from build123d import *

# Parameters (mm, degrees)
BALL_CUT_PATTERN_COUNT      = 3
M3X0_5_TAPPED_HOLE1_REACH   = 23.674
M3X0_5_TAPPED_HOLE1_BORE_R  = 1.25
SET_SCREW_PATTERN_OUTLINE_W = 1.25
SET_SCREW_PATTERN_OUTLINE_H = 2.885095828


# Read off the part's stored shape, not the designer's step: Set Screw Pattern
with BuildPart() as part:
    # Body Sketch → Body Revolve (revolve)
    with BuildSketch(Plane(origin=(-33.219700818, 0, -2.434260963), x_dir=(-1, 0, 0), z_dir=(0, 1, 0)), mode=Mode.PRIVATE) as body_revolve_sk:
        Polygon((-35.719700818, 24.434260963), (-38.269700818, 24.434260963), (-38.269700818, 10.434260963), (-38.169700818, 10.434260963), (-38.169700818, 3.434260963), (-38.269700818, 3.434260963), (-38.269700818, 2.434260963), (-36.769700818, 2.434260963), (-36.769700818, 9.184260963), (-35.719700818, 9.184260963), align=None)
    revolve(body_revolve_sk.sketch.rotate(Axis((0, 0, 0), (0, 0, 1)), 180), axis=Axis((0, 0, 0), (0, 0, 1)))

    # Ball Cut Out Sketch → Ball Cut Revolve (revolve, cut)
    with BuildSketch(Plane(origin=(0, 0, 0), x_dir=(1, 0, 0), z_dir=(0, 1, 0)), mode=Mode.PRIVATE) as ball_cut_revolve_sk:
        with BuildLine():
            Line((4.45, -6), (9.45, -6))
            Line((9.45, -6), (9.45, -4.5))
            Line((9.45, -4.5), (2.95, -4.5))
            ThreePointArc((2.95, -4.5), (3.389339828, -5.560660172), (4.45, -6))
        make_face()
    ball_cut_revolve = revolve(ball_cut_revolve_sk.sketch.rotate(Axis((9.45, 0, 4.5), (-1, 0, 0)), 180), axis=Axis((9.45, 0, 4.5), (-1, 0, 0)), mode=Mode.SUBTRACT)

    # Ball Cut Pattern: Ball Cut Revolve ×3 about axis
    ball_cut_pattern_axis = Axis((0, 0, 0), (0, 0, 1))
    for i in range(1, BALL_CUT_PATTERN_COUNT):
        add(ball_cut_revolve.rotate(ball_cut_pattern_axis, i * 360 / BALL_CUT_PATTERN_COUNT), mode=Mode.SUBTRACT)

    # M3x0.5 Tapped Hole1 bore (on position points) → M3x0.5 Tapped Hole1 (cut, up to next)
    with BuildSketch(Plane(origin=(5.05, 0, 18.5), x_dir=(0, 1, 0), z_dir=(1, 0, 0)), mode=Mode.PRIVATE) as m3x0_5_tapped_hole1_sk1:
        Circle(M3X0_5_TAPPED_HOLE1_BORE_R)
    m3x0_5_tapped_hole1_tool1 = extrude(m3x0_5_tapped_hole1_sk1.sketch, amount=-M3X0_5_TAPPED_HOLE1_REACH, mode=Mode.PRIVATE) & part.part
    add(m3x0_5_tapped_hole1_tool1.solids().sort_by_distance((5.05, 0, 18.5))[0], mode=Mode.SUBTRACT)

    # Set Screw Pattern outline → Set Screw Pattern (revolve, cut)
    with BuildSketch(Plane.YX.offset(-18.5)):
        with Locations((0.625, -3.607452342)):
            Rectangle(SET_SCREW_PATTERN_OUTLINE_W, SET_SCREW_PATTERN_OUTLINE_H)
    revolve(axis=Axis((0, 0, 18.5), (1, 0, 0)), mode=Mode.SUBTRACT)


solid = part.part
Part model, mm, in its own coordinate system. A direction names the side the tool comes from. Give positions to 0.01 mm unless a question says otherwise; leave off trailing zeros. Loops run counter-clockwise (first coordinate to the right, second up) from the corner with the lowest first, then second, coordinate; pieces in that order, holes last. Notation, with made-up numbers: M 14.25,10.25 L 59.25,10.25 A11 cw 59.25,30.25 Z; hole C 72,23.5 d6. An arc over 180 degrees is marked long. Put each result on its own line as item: value. Start each with the question number.
1) Saw through at A-A (y = 0). State how many separate pieces and enclosed holes the cut face has, then the cut area to 3 significant figures.
2) Saw through at D-D (z = 2). List the corners of the cut face in (x, y).
3) 3-axis set-ups, long thin cutter, end or side, ignore diameter. For faces 4 (the flat face through (-2, 2, 6.75)), 5 (the cylindrical face through (-4.817, -1.517, 0.493)), 6 (the cylindrical face through (4.65, -0.45, 3.07)): which of +Z, -Z, +X, -X, +Y, -Y reach the whole face in a straight line?
4) Pull direction X, two halves, no side cores. Call faces 1 (the cylindrical face through (-2.3, 4.1, 6)), 2 (the cylindrical face through (0.64, -4.91, 4.45)), 3 (the cylindrical face through (-3.59, -0.27, 17.28)): +X half, -X half, draft (parallel to the pull), parting line (faces both ways), or undercut.
5) Probe probe 1 along Y at (x, z) = (0, 11); probe 2 along Z at (x, y) = (4.5, 0.75); probe 3 along Z at (x, y) = (4, -1). List the from-to ranges inside material, lowest first.
6) Saw through at C-C (z = 18.5). List the corners of the cut face in (x, y).
7) Flat gauge pins, fed straight in: pin 1 (5 mm diameter, centred on x = -3.5, z = 18.5, fed in from -Y); pin 2 (3 mm diameter, centred on x = 1.5, y = 0.5, fed in from -Z); pin 3 (2 mm diameter, centred on x = 2.5, z = 11.5, fed in from -Y). Where does each tip first touch, or does it go through?
Numbers:
1. separate pieces: 5
1. enclosed holes: 0
1. area: 79.8 mm^2
2. outline: C 0,0 d9.9; hole C 0,0 d7.1
3. face 4: -Z
3. face 5: +Z, -Z
3. face 6: +X
4. face 1: undercut
4. face 2: parting line
4. face 3: draft
5. probe 1: -5.05 to -2.5, 2.5 to 5.05
5. probe 2: 0 to 3.2, 5.8 to 17.5, 19.5 to 22
5. probe 3: 0 to 3.48, 5.52 to 17.75, 19.25 to 22
6. outline: M -4.89,-1.25 A5.05 ccw 4.89,-1.25 L 2.17,-1.25 A2.5 cw -2.17,-1.25 Z; M -4.89,1.25 L -2.17,1.25 A2.5 cw 2.17,1.25 L 4.89,1.25 A5.05 ccw Z
7. pin 1: y = -4.95
7. pin 2: z = 6.75
7. pin 3: y = -4.82
